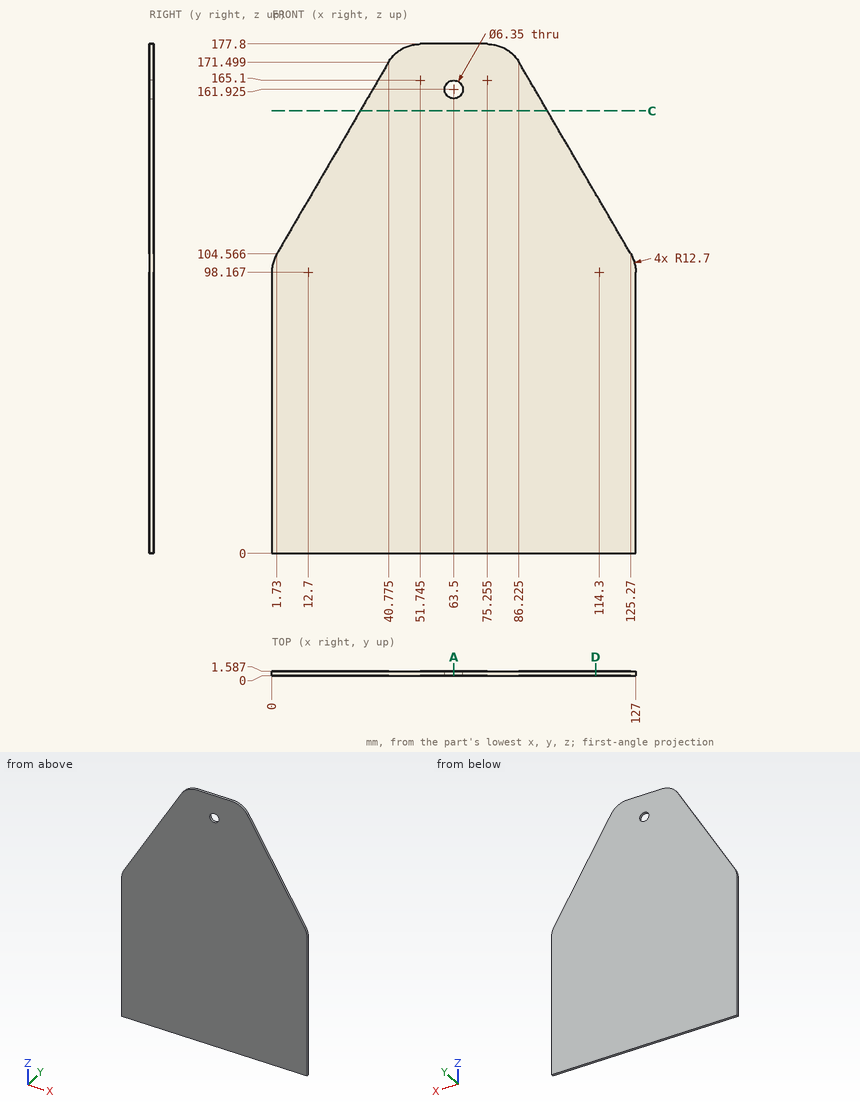
Part print with two shaded views. Sizes in mm from the minimum x, y, z corner. Coordinates: 2 decimals unless noted, no trailing zeros. Write each loop counter-clockwise with the first axis right and the second up, starting at its lowest first coordinate (ties: lowest second). Pieces come first, ordered by that corner, then holes. Notation, with made-up numbers: (26.25, -40) -> (72.25, -40) arc R25 ccw to (72.25, -17) -> close; hole circle Ø7 at (77.5, 25.5). An arc over 180 degrees is marked (long way). Return JSON: item names as keys, results as strings. Group by question number.
Q1. Drill centre lines: line 1 (Z direction, x = 64.5, y = 0.65); line 2 (Z direction, x = 22.5, y = 0.2) (1 decimal); line 3 (Z direction, x = 21.5, y = 0.3) (1 decimal). Where is each one in solid material? Low to high.
Q2. Cut at A-A, the plane x = 63.5. Give the cut face in (y, z).
Q3. Cut at C-C, the plane z = 154.5. Give the cut face in (x, y), then the cut area to 3 significant figures.
Q4. Cut at D-D, the plane x = 113. Give the cut face in (y, z).
Returned:
{
 "1": {"line 1": "z = 0 to 158.91, 164.94 to 177.8", "line 2": "z = 0 to 140.2", "line 3": "z = 0 to 138.5"},
 "2": {"outline": "(0, 0) -> (1.59, 0) -> (1.59, 158.75) -> (0, 158.75) -> close; (0, 165.1) -> (1.59, 165.1) -> (1.59, 177.8) -> (0, 177.8) -> close"},
 "3": {"outline": "(30.86, 0) -> (96.14, 0) -> (96.14, 1.59) -> (30.86, 1.59) -> close", "area": "104 mm2"},
 "4": {"outline": "(0, 0) -> (1.59, 0) -> (1.59, 125.6) -> (0, 125.6) -> close"}
}
